Answer from the drawing. Dimensions are ordinates in mm from the lowest x, y and z of the part. A direction names the side the tool comes from. Give positions to 0.01 mm unless a question says otherwise; leave off trailing zeros. Order: outer loops, then holes, each group sorted by start corner. A loop starts at its lowest first (then second) coordinate and runs counter-clockwise, first axis right, second up. Notation, with made-up numbers: (58.25, 81.5) - (106.25, 81.5) arc R23 cw to (106.25, 89.5) - close; hole circle Ø9 at (-16.5, 5). An arc over 180 degrees is marked (long way). Write each question's results on one line, items separated by ' | '.
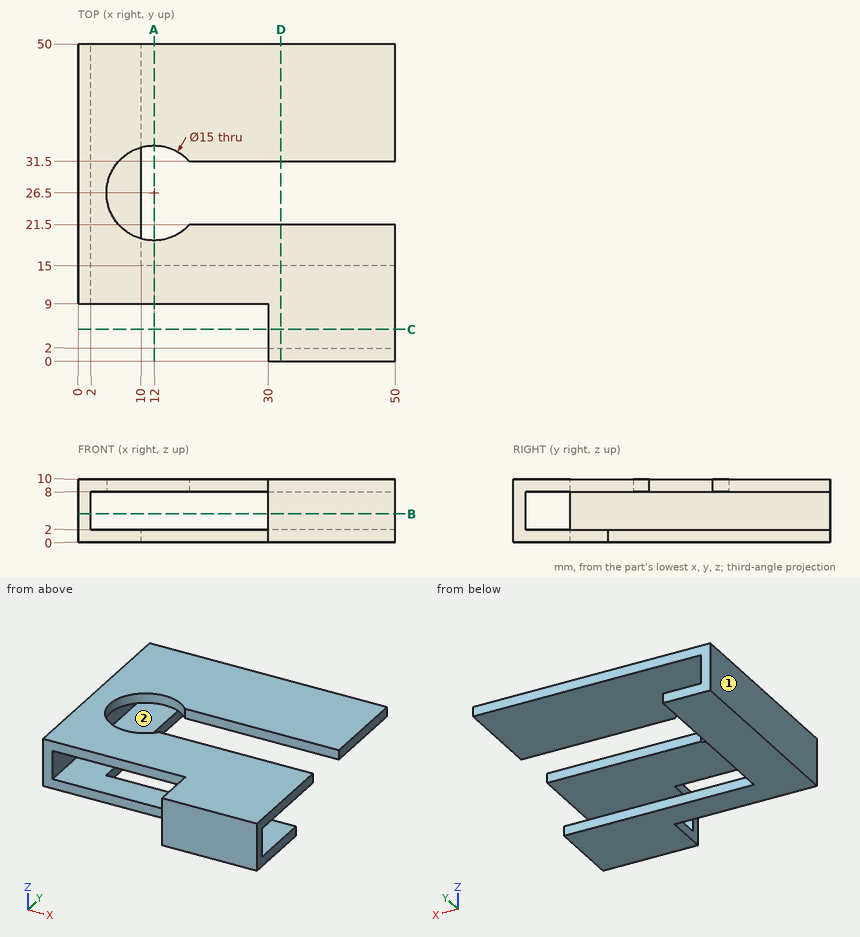
1. A cutting plane is placed at A-A, the plane x = 12. Write down the section's boundary in (y, z), then the cut area to 3 significant figures.
Answer list:
outline: (9, 0) - (15, 0) - (15, 2) - (9, 2) - close; (9, 8) - (19, 8) - (19, 10) - (9, 10) - close; (34, 8) - (50, 8) - (50, 10) - (34, 10) - close | area: 64.0 mm^2
2. A cutting plane is placed at C-C, the plane y = 5. Write down the section's boundary in (x, z), then the cut area to 3 significant figures.
Answer list:
outline: (30, 0) - (50, 0) - (50, 2) - (30, 2) - close; (30, 8) - (50, 8) - (50, 10) - (30, 10) - close | area: 80.0 mm^2
3. A cutting plane is placed at B-B, the plane z = 4.5. Write down the section's boundary in (x, y).
Answer list:
outline: (0, 9) - (2, 9) - (2, 50) - (0, 50) - close; (30, 0) - (50, 0) - (50, 2) - (30, 2) - close
4. Straight lines are drawn through the part: line 1 (Z direction, x = 7, y = 13); line 2 (Y direction, x = 12, z = 9.55); line 3 (X direction, y = 26.5, z = 9.65). For each, find the intervals that lie inside material, in ascending order. Write a range as [from, to].
Answer list:
line 1: [0, 2], [8, 10] | line 2: [9, 19], [34, 50] | line 3: [0, 4.5]
5. Given P1, Ø3, axis at x = 43.5, z = 2.5, coming from the -Y side; P2, Ø5, axis at x = 43.5, z = 5, coming from the +Y side; P3, Ø1.6, axis at y = 39.5, z = 0.5, coming from the +X side; P4, Ø3, axis at x = 12.5, z = 5.5, coming from the -Y side, each flat-ended and moving along its own axis, determine where each tip first touches the part or whether it passes through.
Answer list:
P1: y = 0 | P2: y = 2 | P3: x = 10 | P4: through
6. A tool of negligible diameter and unlimited length cuts with its end or side. For the marked faces 1 and 2, from which of +Z, -Z, +X, -X, +Y, -Y can it reach the whole face along a straight path? Write none if from no direction.
Answer list:
face 1: +Z, -Z, -X, +Y, -Y | face 2: +X, +Y
7. A cutting plane is placed at D-D, the plane x = 32. Write down the section's boundary in (y, z).
Answer list:
outline: (0, 0) - (15, 0) - (15, 2) - (2, 2) - (2, 8) - (21.5, 8) - (21.5, 10) - (0, 10) - close; (31.5, 8) - (50, 8) - (50, 10) - (31.5, 10) - close
